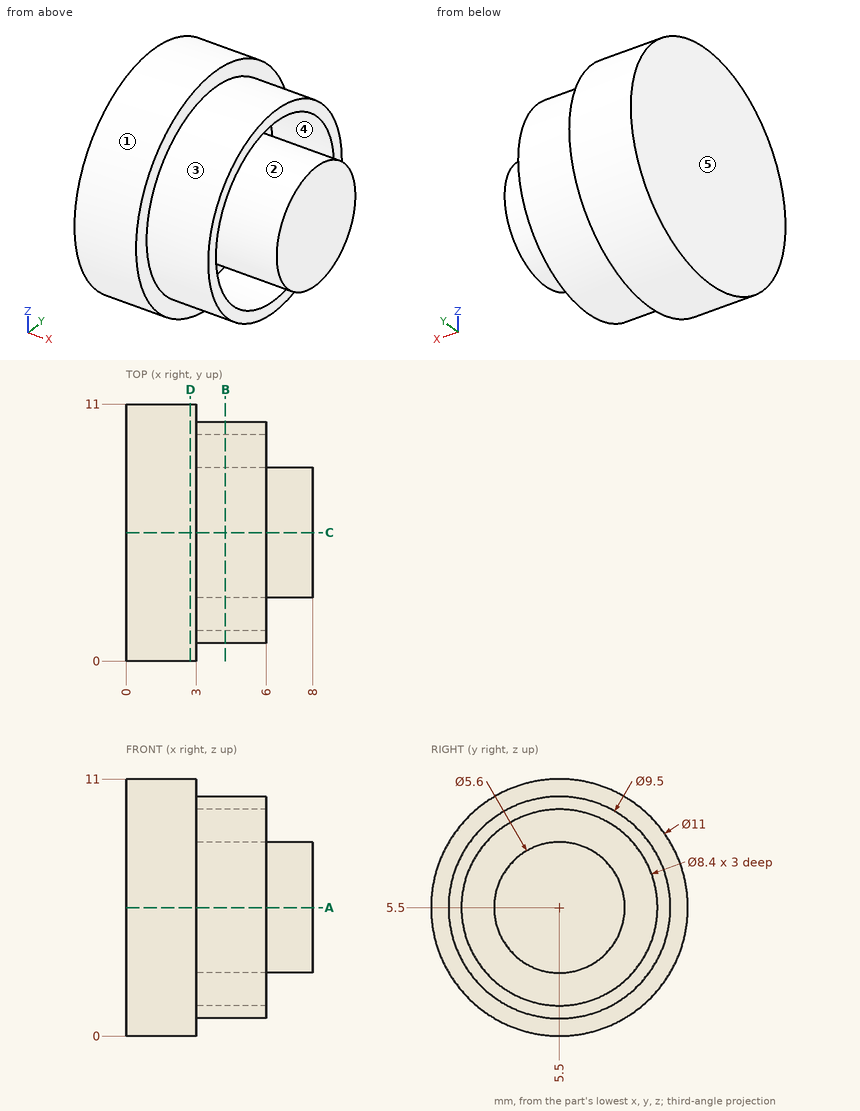
Study the drawing (mm; zero at the part's minimum x, y, z) and answer. A direction names the side the tool comes from. Coordinates: 2 decimals unless noted, no trailing zeros. Write each loop counter-clockwise with the first axis right and the second up, starting at its lowest first coordinate (ties: lowest second). Pieces come first, ordered by that corner, then holes. Notation, with made-up numbers: (83.25, -32.5) -> (110.25, -32.5) arc R21 cw to (110.25, -23.5) -> close; hole circle Ø1 at (-2, -27.75). An arc over 180 degrees is marked (long way). Write each question's results on one line, items separated by ' | '. Start each with the question number.
1) Flat-ended cylindrical pins translate along their axes: pin 1 Ø1 at (y, z) = (3.5, 2.5) entering from -X; pin 2 Ø3 at (x, z) = (6, 7) entering from -Y. Find the tip coordinate at first contact, or state that the pin passes through.
2) Straight lines are drawn through the part: probe 1 along Z at (x, y) = (3.85, 5.5); probe 2 along Y at (x, z) = (4.75, 3); probe 3 along Z at (x, y) = (4.25, 3.75). For each, find the intervals that lie inside material, in ascending order.
3) A tool of negligible diameter and unlimited length cuts with its end or side. For the marked faces 1 and 2, from which of +Z, -Z, +X, -X, +Y, -Y can it reach the whole face along a straight path? Write none if from no direction.
4) For a pull along Y with two mould halves and no side action, classify the marked faces 3, 4 and 5 as +Y half, -Y half, draft (parallel to the pull), parting line (faces both ways), or undercut.
5) A cutting plane is placed at B-B (x = 4.25). Determine the outline of the cut face in (y, z), then the cut area to 3 significant figures.
6) A cutting plane is placed at D-D (x = 2.75). Determine the outline of the cut face in (y, z).
7) A cutting plane is placed at A-A (z = 5.5). Determine the outline of the cut face in (x, y).
Values follow:
1) pin 1: x = 0 | pin 2: y = 0.75
2) probe 1: 0.75 to 1.3, 2.7 to 8.3, 9.7 to 10.25 | probe 2: 1.46 to 2.13, 4.24 to 6.76, 8.87 to 9.54 | probe 3: 1.08 to 1.68, 3.31 to 7.69, 9.32 to 9.92
3) face 1: +X, -X | face 2: +X
4) face 3: parting line | face 4: undercut | face 5: draft
5) outline: circle Ø9.5 at (5.5, 5.5); circle Ø5.6 at (5.5, 5.5); hole circle Ø8.4 at (5.5, 5.5) | area: 40.1 mm²
6) outline: circle Ø11 at (5.5, 5.5)
7) outline: (0, 0) -> (3, 0) -> (3, 0.75) -> (6, 0.75) -> (6, 1.3) -> (3, 1.3) -> (3, 2.7) -> (8, 2.7) -> (8, 8.3) -> (3, 8.3) -> (3, 9.7) -> (6, 9.7) -> (6, 10.25) -> (3, 10.25) -> (3, 11) -> (0, 11) -> close
